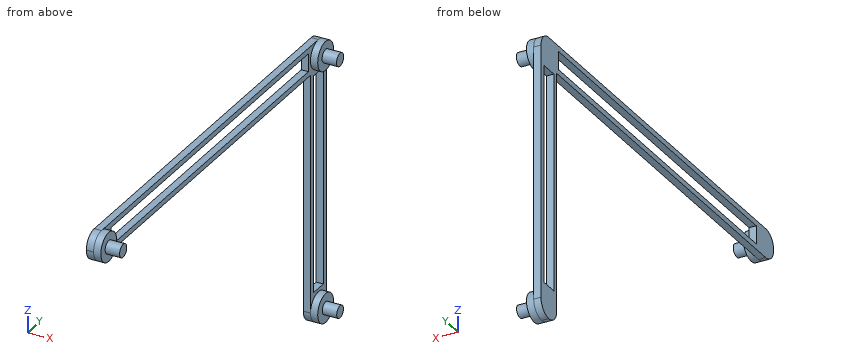
from build123d import *

# Parameters (mm, degrees)
SKETCH1_W           = 4
SKETCH1_H           = 54.9
SKETCH1_W_2         = 38.9
SKETCH1_H_2         = 4
BOSS_EXTRUDE1_DEPTH = 1
SKETCH2_R           = 2
BOSS_EXTRUDE2_DEPTH = 1
SKETCH3_R           = 0.9
SKETCH3_R_2         = 0.85
BOSS_EXTRUDE3_DEPTH = 2
SKETCH4_W           = 30
SKETCH4_H           = 2.5
SKETCH4_W_2         = 2.5
SKETCH4_H_2         = 50
CUT_EXTRUDE1_DEPTH  = 1
FILLET1_R           = 2


with BuildPart() as part:
    # Sketch1 → Boss-Extrude1 (new body)
    with BuildSketch(Plane(origin=(0, 0, 0), x_dir=(0, 0, -1), z_dir=(1, 0, 0))):
        with Locations((-17.45, -29.45)):
            Rectangle(SKETCH1_W, SKETCH1_H)
        Rectangle(SKETCH1_W_2, SKETCH1_H_2)
    extrude(amount=BOSS_EXTRUDE1_DEPTH)

    # Sketch2 → Boss-Extrude2 (add)
    with BuildSketch(Plane(origin=(1, 0, 0), x_dir=(0, 0, -1), z_dir=(1, 0, 0))):
        with Locations(Location((-17.45, 0, 0), (0, 0, 180))):
            Circle(SKETCH2_R)
        with Locations((17.45, 0)):
            Circle(SKETCH2_R)
        with Locations((-17.45, -54.9)):
            Circle(SKETCH2_R)
    extrude(amount=BOSS_EXTRUDE2_DEPTH)

    # Sketch3 → Boss-Extrude3 (add)
    with BuildSketch(Plane(origin=(2, 0, 0), x_dir=(0, 0, -1), z_dir=(1, 0, 0))):
        with Locations((-17.45, 0)):
            Circle(SKETCH3_R)
        with Locations((17.45, 0)):
            Circle(SKETCH3_R_2)
        with Locations((-17.45, -54.9)):
            Circle(SKETCH3_R)
    extrude(amount=BOSS_EXTRUDE3_DEPTH)

    # Sketch4 → Cut-Extrude1 (cut)
    with BuildSketch(Plane(origin=(1, 0, 0), x_dir=(0, 0, -1), z_dir=(1, 0, 0))):
        Rectangle(SKETCH4_W, SKETCH4_H)
        with Locations((-17.45, -27.5)):
            Rectangle(SKETCH4_W_2, SKETCH4_H_2)
    extrude(amount=-CUT_EXTRUDE1_DEPTH, mode=Mode.SUBTRACT)

    # Fillet1
    fillet1_edges = [part.edges().sort_by_distance(p)[0] for p in [
        (0.5, 2, 19.45),
        (0.5, 2, -19.45),
        (0.5, -2, -19.45),
        (0.5, -56.9, 15.45),
        (0.5, -56.9, 19.45),
    ]]
    fillet(fillet1_edges, radius=FILLET1_R - 0.0001)  # a hair under: the kernel refuses the full size


solid = part.part
Read the model definition and answer for the solid it produces. Units are mm, in the model's axes. Round coordinates to 2 decimals unless told otherwise and drop trailing zeros. Write each loop counter-clockwise with the first axis right and the second up, starting at its lowest first coordinate (ties: lowest second). Pieces come first, ordered by that corner, then holes. Notation, with made-up numbers: (-12, 51.5) - (-8, 51.5) arc R36 ccw to (-8, 88.5) - close; hole circle Ø11 at (-22, 8.5). An arc over 180 degrees is marked (long way). Use a Markdown table: item, result.
(1) The part is cut by section B-B (z = 0). Write down the section's boundary in (x, y), then the cut area to 3 significant figures.
Reported:
| item | result |
|---|---|
| outline | (0, -2) - (1, -2) - (1, -1.25) - (0, -1.25) - close; (0, 1.25) - (1, 1.25) - (1, 2) - (0, 2) - close |
| area | 1.50 mm2 |
(2) Each of these flat-tipped pins is pushed along its axis until it touches: pin 1 Ø1.2 at (y, z) = (-54, 17) entering from +X; pin 2 Ø0.5 at (x, y) = (0.5, -28) entering from -Z; pin 3 Ø0.5 at (x, z) = (0.5, 2.5) entering from -Y; pin 4 Ø0.6 at (y, z) = (-0.5, -19) entering from +X. Where does it stop, or does it pass through?
Reported:
| item | result |
|---|---|
| pin 1 | x = 4 |
| pin 2 | z = 15.45 |
| pin 3 | y = -2 |
| pin 4 | x = 2 |
(3) The part is cut by section C-C (x = 3.35). Write down the section's boundary in (y, z), then the cut area to 3 significant figures.
Reported:
| item | result |
|---|---|
| outline | circle Ø1.8 at (-54.9, 17.45); circle Ø1.8 at (0, 17.45); circle Ø1.7 at (0, -17.45) |
| area | 7.36 mm2 |
(4) The part is cut by section A-A (y = -35.5). Write down the section's boundary in (x, z), then the cut area to 3 significant figures.
Reported:
| item | result |
|---|---|
| outline | (0, 15.45) - (1, 15.45) - (1, 16.2) - (0, 16.2) - close; (0, 18.7) - (1, 18.7) - (1, 19.45) - (0, 19.45) - close |
| area | 1.50 mm2 |
(5) Straight lines are drawn through the part: line 1 along Y through (x, z) = (0.3, -9.5); line 2 along Z through (x, y) = (0.25, -39.5); line 3 along X through (y, z) = (-36, 16). For each, find the intervals that lie inside material, in ascending order. Write a range as [from, to].
Reported:
| item | result |
|---|---|
| line 1 | [-2, -1.25], [1.25, 2] |
| line 2 | [15.45, 16.2], [18.7, 19.45] |
| line 3 | [0, 1] |
